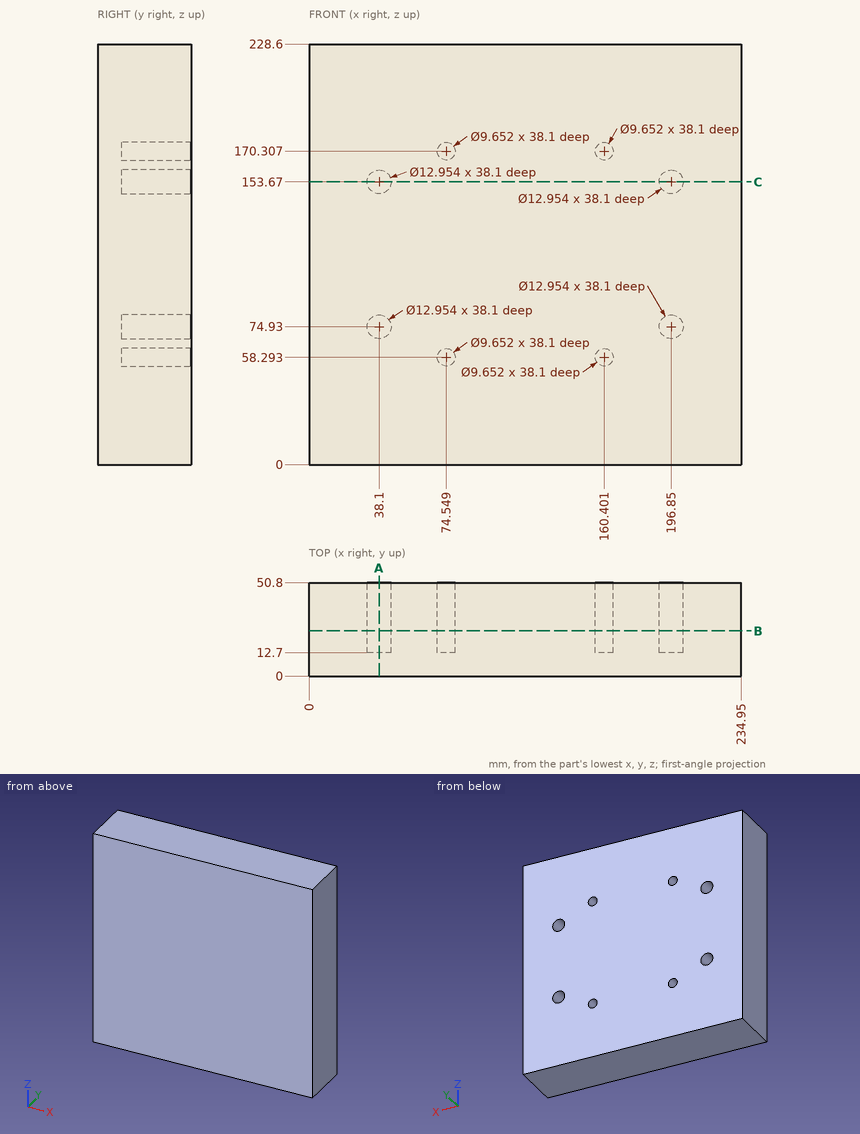
Study the drawing (mm; zero at the part's minimum x, y, z) and answer. Round coordinates to 2 decimals unless told otherwise and drop trailing zeros. Write each loop counter-clockwise with the first axis right and the second up, starting at its lowest first coordinate (ties: lowest second). Pieces come first, ordered by that corner, then holes. Notation, with made-up numbers: (33, 18) -> (42, 18) arc R22 cw to (42, 33) -> close; hole circle Ø8 at (53, -30). An arc over 180 degrees is marked (long way). Answer as CSV lines item,"result". Start each with the question number.
(1) The part is cut by section C-C, the plane z = 153.67. Give the vertices of the cut face in (x, y), then the cut area to 3 significant figures.
(2) The part is cut by section A-A, the plane x = 38.1. Give the vertices of the cut face in (y, z), then the cut area to 3 significant figures.
(3) Find the intervals of material crossed by probe 1 along X at (y, z) = (43, 153); probe 2 along Z at (x, y) = (196, 36); probe 3 along Z at (x, y) = (72, 14), in increasing order.
(4) This flat-tipped pin is pushed along its axis until it touches: pin 1 (7.5 mm diameter, centred on x = 160.401, z = 170.307, fed in from +Y). Where does it stop, or does it pass through?
(5) The part is cut by section B-B, the plane y = 24.5. Give the number of separate pieces and of enclosed holes in the cut face, then the cut area to 3 significant figures.
Output values:
1,outline,"(0, 0) -> (234.95, 0) -> (234.95, 50.8) -> (203.33, 50.8) -> (203.33, 12.7) -> (190.37, 12.7) -> (190.37, 50.8) -> (44.58, 50.8) -> (44.58, 12.7) -> (31.62, 12.7) -> (31.62, 50.8) -> (0, 50.8) -> close"
1,area,"10,900 mm²"
2,outline,"(0, 0) -> (50.8, 0) -> (50.8, 68.45) -> (12.7, 68.45) -> (12.7, 81.41) -> (50.8, 81.41) -> (50.8, 147.19) -> (12.7, 147.19) -> (12.7, 160.15) -> (50.8, 160.15) -> (50.8, 228.6) -> (0, 228.6) -> close"
2,area,"10,600 mm²"
3,probe 1,"x = 0 to 31.66, 44.54 to 190.41, 203.29 to 234.95"
3,probe 2,"z = 0 to 68.51, 81.35 to 147.25, 160.09 to 228.6"
3,probe 3,"z = 0 to 54.2, 62.39 to 166.21, 174.4 to 228.6"
4,pin 1,"stops at y = 12.7"
5,separate pieces,"1"
5,enclosed holes,"8"
5,area,"52,900 mm²"
